```python
from build123d import *

# Parameters (mm, degrees)
F0_W           = 60
F0_H           = 60
F1_DEPTH       = 3
F2_R           = 20
F3_DEPTH       = 147
F4_R           = 5
F6_D           = 5
F6_CSINK_D     = 10
F6_CSINK_ANGLE = 90
F7_R           = 1


with BuildPart() as f1:
    # F0 (on Top) → F1 (new body)
    with BuildSketch(Plane.XY):
        Rectangle(F0_W, F0_H)
    extrude(amount=-F1_DEPTH)

    # F2 (on face) → F3 (join)
    with BuildSketch(Plane(origin=(0, 0, -3), x_dir=(1, 0, 0), z_dir=(0, 0, -1))):
        Circle(F2_R)
    extrude(amount=F3_DEPTH)

    # F4
    f4_edges = [f1.edges().sort_by_distance(p)[0] for p in [
        (-30, -30, -1.5),
        (30, -30, -1.5),
        (30, 30, -1.5),
        (-30, 30, -1.5),
    ]]
    fillet(f4_edges, radius=F4_R)

    # F6 (through all)
    with Locations(Plane(origin=(0, 0, -3), x_dir=(1, 0, 0), z_dir=(0, 0, -1))):
        with Locations((-22, 22), (22, 22), (22, -22), (-22, -22)):
            CounterSinkHole(F6_D / 2, F6_CSINK_D / 2, counter_sink_angle=F6_CSINK_ANGLE)

    # F7
    f7_edges = [f1.edges().sort_by_distance(p)[0] for p in [
        (-20, 0, -150),
    ]]
    fillet(f7_edges, radius=F7_R)


solid = f1.part
```
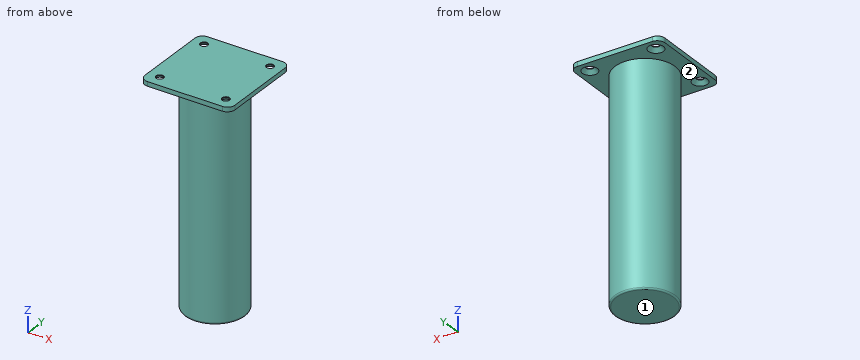
Input: part model. Units: mm. Frame: model coordinates. Face numbers are marked on the shaded views. A direction names the side the tool comes from. Round coordinates to 2 decimals unless told otherwise and drop trailing zeros. Order: outer loops, then holes, each group sorted by start corner. A loop starts at its lowest first (then second) coordinate and runs counter-clockwise, first axis right, second up. Notation, with made-up numbers: (-40, 30) - (-22, 30) arc R14 cw to (-22, 34) - close; hole circle Ø2 at (79.25, 79). An arc over 180 degrees is marked (long way). Answer in a Markdown table with one row per item.
Item 1: Section query C-C (z = -26.5). Return the cut outline in (x, y), then the cut area to 3 significant figures.
Model answer:
| item | result |
|---|---|
| outline | circle Ø40 at (0, 0) |
| area | 1,260 mm² |
Item 2: Section query A-A (x = -22). Return the cut outline in (y, z), then the cut area to 4 significant figures.
Model answer:
| item | result |
|---|---|
| outline | (-30, -3) - (-27, -3) - (-24.5, -0.5) - (-24.5, 0) - (-30, 0) - close; (-19.5, -0.5) - (-17, -3) - (17, -3) - (19.5, -0.5) - (19.5, 0) - (-19.5, 0) - close; (24.5, -0.5) - (27, -3) - (30, -3) - (30, 0) - (24.5, 0) - close |
| area | 137.5 mm² |
Item 3: Section query B-B (y = 0). Return the cut outline in (x, z), then the cut area to 3 significant figures.
Model answer:
| item | result |
|---|---|
| outline | (-30, -3) - (-20, -3) - (-20, -149) arc R1 ccw to (-19, -150) - (19, -150) arc R1 ccw to (20, -149) - (20, -3) - (30, -3) - (30, 0) - (-30, 0) - close |
| area | 6,060 mm² |
Item 4: Reachability of the marked faces 1 and 2 from +Z, -Z, +X, -X, +Y, -Y: full face, straight path, thin tool, end or side. Return the list, or none.
Model answer:
| item | result |
|---|---|
| face 1 | -Z, +X, -X, +Y, -Y |
| face 2 | -Z |
Item 5: Line query: line 1 (Y direction, x = 22, z = -0.05); line 2 (Z direction, x = 11, y = -26.5). Output: solid intervals per line, ascending.
Model answer:
| item | result |
|---|---|
| line 1 | y = -30 to -24.5, -19.5 to 19.5, 24.5 to 30 |
| line 2 | z = -3 to 0 |
Item 6: Pin query (flat end, axial travel): pin 1 (2 mm diameter, centred on y = -14, z = -56, fed in from +X); pin 2 (2 mm diameter, centred on x = -1.5, z = -134.5, fed in from +Y); pin 3 (10 mm diameter, centred on y = -23.5, z = -66.5, fed in from -X). Return the tip coordinate at first contact, or that it passes through.
Model answer:
| item | result |
|---|---|
| pin 1 | stops at x = 15.2 |
| pin 2 | stops at y = 19.99 |
| pin 3 | stops at x = -7.6 |
